```python
from build123d import *

# Parameters (mm, degrees)
BOSS_EXTRUDE1_DEPTH = 25.4
SKETCH2_W           = 38.862
SKETCH2_H           = 38.862
CUT_EXTRUDE1_DEPTH  = 303.885239179
FILLET1_R           = 6.35
FILLET2_R           = 3.175
SKETCH3_R           = 4.191
CUT_EXTRUDE2_DEPTH  = 314.875552812
SKETCH4_R           = 4.191
CUT_EXTRUDE3_DEPTH  = 25.4


with BuildPart() as part:
    # Sketch1 → Boss-Extrude1 (new body)
    with BuildSketch(Plane.XY):
        Polygon((0, 0), (0, 12.7), (50.8, 12.7), (88.9, -20.510228633), (152.4, -260.515926793), (38.018659419, -260.515926793), (38.018659419, -190.696503564), (30.48, -85.763926793), (0, -85.763926793), (0, -73.152260366), (38.018659419, -73.152260366), (38.018659419, 0), align=None)
    extrude(amount=BOSS_EXTRUDE1_DEPTH)

    # Sketch2 → Cut-Extrude1 (cut, through all)
    with BuildSketch(Plane(origin=(0, 0, 0), x_dir=(-1, 0, 0), z_dir=(0, 0, -1))):
        with Locations((-82.955564704, -163.868926793)):
            Rectangle(SKETCH2_W, SKETCH2_H)
    extrude(amount=-CUT_EXTRUDE1_DEPTH, mode=Mode.SUBTRACT)

    # Fillet1
    # the kernel refuses this fillet: 6.35 mm, written as the material it adds along each edge
    with BuildSketch(Plane(origin=(38.018659419, -190.696503564, 0), x_dir=(0, -1, 0), z_dir=(0, 0, 1))) as fillet1_piece_1:
        with BuildLine():
            CenterArc((FILLET1_R * 0.0358752122725, -FILLET1_R), FILLET1_R, 90, 4.109234206)
            Line((-FILLET1_R * 0.0357829859603, -FILLET1_R * 0.00257075307266), (0, 0))
            Line((0, 0), (FILLET1_R * 0.0358752122725, 0))
        make_face()
    extrude(amount=25.4)
    with BuildSketch(Plane(origin=(30.48, -85.763926793, 0), x_dir=(-1, 0, 0), z_dir=(0, 0, 1))) as fillet1_piece_2:
        with BuildLine():
            CenterArc((FILLET1_R * 0.930734490318, FILLET1_R), FILLET1_R, 184.109234206, 85.890765794)
            Line((-FILLET1_R * 0.0666947566093, FILLET1_R * 0.928341801767), (0, 0))
            Line((0, 0), (FILLET1_R * 0.930734490318, 0))
        make_face()
    extrude(amount=25.4)
    # the kernel refuses this fillet: 6.35 mm, written as the material it takes off along each edge
    with BuildSketch(Plane(origin=(50.8, 12.7, -5.947635314), x_dir=(-1, 0, 0), z_dir=(0, 0, 1))) as fillet1_2_piece_1:
        with BuildLine():
            CenterArc((FILLET1_R * 0.374654193004, FILLET1_R), FILLET1_R, 228.922654606, 41.077345394)
            Line((-FILLET1_R * 0.282423044355, FILLET1_R * 0.246176742103), (0, 0))
            Line((0, 0), (FILLET1_R * 0.374654193004, 0))
        make_face()
    extrude(amount=37.295270628, mode=Mode.SUBTRACT)
    with BuildSketch(Plane(origin=(88.9, -20.510228633, -4.869092834), x_dir=(-0.7538232578965339, 0.6570772373581782, 0), z_dir=(0, 0, 1))) as fillet1_2_piece_2:
        with BuildLine():
            CenterArc((FILLET1_R * 0.306714509228, FILLET1_R), FILLET1_R, 235.896927034, 34.103072966)
            Line((-FILLET1_R * 0.253968896194, FILLET1_R * 0.171969735526), (0, 0))
            Line((0, 0), (FILLET1_R * 0.306714509228, 0))
        make_face()
    extrude(amount=35.138185668, mode=Mode.SUBTRACT)

    # Fillet2
    fillet2_edges = [part.edges().sort_by_distance(p)[0] for p in [
        (63.524564704, -144.437926793, 12.7),
        (63.524564704, -183.299926793, 12.7),
        (102.386564704, -183.299926793, 12.7),
        (102.386564704, -144.437926793, 12.7),
    ]]
    fillet(fillet2_edges, radius=FILLET2_R)

    # Sketch3 → Cut-Extrude2 (cut, through all)
    with BuildSketch(Plane(origin=(0, 12.7, 0), x_dir=(1, 0, 0), z_dir=(0, 1, 0))):
        with Locations(Location((11.684, -12.7, 0), (0, 0, 270))):
            Circle(SKETCH3_R)
    extrude(amount=-CUT_EXTRUDE2_DEPTH, mode=Mode.SUBTRACT)

    # Sketch4 → Cut-Extrude3 (cut)
    with BuildSketch(Plane.XZ.offset(260.515926793)):
        with Locations((139.7, 12.7)):
            Circle(SKETCH4_R)
        with Locations((63.5, 12.7)):
            Circle(SKETCH4_R)
    extrude(amount=-CUT_EXTRUDE3_DEPTH, mode=Mode.SUBTRACT)


solid = part.part
```
Here's how the part is built. I have some questions about the finished solid (model axes, mm). A direction names the side the tool comes from. Give positions to 0.01 mm unless a question says otherwise; leave off trailing zeros. Order: outer loops, then holes, each group sorted by start corner. A loop starts at its lowest first (then second) coordinate and runs counter-clockwise, first axis right, second up. Notation, with made-up numbers: (20, 29) - (52, 29) arc R21 ccw to (52, 52) - close; hole circle Ø1 at (16, -19). An arc over 180 degrees is marked (long way). Answer as a JSON object with one key per item and string values. Group by question number.
Item 1: For P1, Ø5, axis at x = 11.684, z = 12.7, coming from the -Y side; P2, Ø11, axis at x = 11.684, z = 12.7, coming from the -Y side; P3, Ø12.5, axis at x = 84, z = 13, coming from the +Y side; P4, Ø7.5, axis at y = -235, z = 19, coming from the -X side, each with a flat end and sliding along its axis, tell me the tip position at first contact or that it passes through.
Item 2: If we section it at D-D on y = -125: Please give me the cut outline in (x, z), and give its area (3 significant figures).
Item 3: Please list where these lines run through material, in increasing order: probe 1 along Z at (x, y) = (63, -246); probe 2 along X at (y, z) = (-148.5, 3.5); probe 3 along X at (y, z) = (-77.5, 12.7) (3 decimals).
Item 4: If we section it at C-C on x = 139.7: Please give me the cut outline in (y, z), and give its area (3 significant figures).
Item 5: If we section it at A-A on z = 12.7: Give the number of separate pieces and of enclosed holes in the cut face, and give its area (3 significant figures).
Item 6: Which directions (+Z, -Z, +X, -X, +Y, -Y) give clear straight access to the entire face, cutting with the end or side of a thin tool? Please do faces 5 (the flat face through (102.387, -164, 13)), 6 (the flat face through (0, 6, 13)), 7 (the flat face through (69.769, -3.834, 12.522)), 8 (the flat face through (19, -73.152, 13)), 9 (the flat face through (140, -235.116, 13)).
Item 7: If we section it at B-B on y = -161: Please give me the cut outline in (x, z), and give its area (3 significant figures).
Item 8: If we mould it in two halves opening along Z, with no side actions, what happens to faces 1 (the flat face through (58, -156, 0)), 2 (the cylindrical face through (67.497, -247.994, 13.959)), 3 (the flat face through (15.2, -85.764, 15.3)), 4 (the cylindrical face through (15.84, -79.37, 12.15))? For each: pulls with the +Z half, pulls with the -Z half, needs draft (parallel to the pull), parting line crosses it, or undercut.
Result set:
{
 "1": {"P1": "through", "P2": "y = -85.76", "P3": "y = -10.79", "P4": "x = 38.02"},
 "2": {"outline": "(33.3, 0) - (116.55, 0) - (116.55, 25.4) - (33.3, 25.4) - close", "area": "2,110 mm²"},
 "3": {"probe 1": "0 to 8.54, 16.86 to 25.4", "probe 2": "34.99 to 63.52, 102.39 to 122.76", "probe 3": "0 to 7.493, 15.875 to 103.978"},
 "4": {"outline": "(-260.52, 0) - (-212.51, 0) - (-212.51, 25.4) - (-260.52, 25.4) - (-260.52, 16.89) - (-235.12, 16.89) - (-235.12, 8.51) - (-260.52, 8.51) - close", "area": "1,010 mm²"},
 "5": {"separate pieces": "3", "enclosed holes": "1", "area": "20,100 mm²"},
 "6": {"face 5": "+Z, -Z", "face 6": "+Z, -Z, -X, +Y, -Y", "face 7": "+Z, -Z, +X, +Y", "face 8": "+Z, -Z, -X", "face 9": "-Y"},
 "7": {"outline": "(35.89, 0) - (63.52, 0) - (63.52, 25.4) - (35.89, 25.4) - close; (102.39, 0) - (126.07, 0) - (126.07, 25.4) - (102.39, 25.4) - close", "area": "1,300 mm²"},
 "8": {"face 1": "pulls with the -Z half", "face 2": "undercut", "face 3": "needs draft", "face 4": "undercut"}
}
